```python
from build123d import *

# Parameters (mm, degrees)
F0_W         = 3.3528
F0_H         = 2.5146
F0_R         = 0.80645
F0_W_2       = 6.35
F0_H_2       = 10.7442
F1_DEPTH     = 3.048
F2_W         = 2.54
F2_H         = 10.7442
F2_W_2       = 22.86
F2_H_2       = 7.9502
F3_DEPTH     = 1.27
F4_W         = 6.35
F4_H         = 5.715
F5_DEPTH     = 2.54
F6_R         = 0.79375
F7_DEPTH     = 10.7452
F8_DEPTH     = 0.508
F9_W         = 3.81
F9_H         = 2.5146
F10_DEPTH    = 0.762
F11_T1_DEPTH = 10.445747458
F11_T3_DEPTH = 10.445747458
F11_T5_DEPTH = 12.6746
F11_T7_DEPTH = 12.6746
F12_R        = 0.381
F13_DEPTH    = 1.397


# Not quite as in the source:
# - a fillet or chamfer that OpenCascade refuses, or shapes differently, is made with other operations: its cross-section is extruded or revolved along the edge and cut away or added
# - a feature names something its author has since deleted; it is built from what else it names


with BuildPart() as f1:
    # F0 (on Top) → F1 (new body)
    with BuildSketch(Plane.XY):
        with Locations((-12.8524, 4.1148)):
            Rectangle(F0_W, F0_H)
        with Locations((-12.8524, -4.1148)):
            Rectangle(F0_W, F0_H)
        Polygon((14.478, -5.3721), (14.478, 5.3721), (-11.176, 5.3721), (-11.176, 2.8575), (-11.176, -2.8575), (-11.176, -5.3721), align=None)
        with Locations((-7.366, 0)):
            Circle(F0_R, mode=Mode.SUBTRACT)
        with BuildLine():
            ThreePointArc((-1.7885716042, 1.644670926), (-2.2375844102, 2.728683732), (-1.1535716042, 2.279670926))
            Line((-1.1535716042, 2.279670926), (1.1535716042, 2.279670926))
            ThreePointArc((1.1535716042, 2.279670926), (2.2375844102, 2.728683732), (1.7885716042, 1.644670926))
            Line((1.7885716042, 1.644670926), (1.7885716042, 0.635))
            ThreePointArc((1.7885716042, 0.635), (2.4235716042, 0), (1.7885716042, -0.635))
            Line((1.7885716042, -0.635), (1.7885716042, -1.644670926))
            ThreePointArc((1.7885716042, -1.644670926), (2.2375844102, -2.728683732), (1.1535716042, -2.279670926))
            Line((1.1535716042, -2.279670926), (-1.1535716042, -2.279670926))
            ThreePointArc((-1.1535716042, -2.279670926), (-2.2375844102, -2.728683732), (-1.7885716042, -1.644670926))
            Line((-1.7885716042, -1.644670926), (-1.7885716042, -0.635))
            ThreePointArc((-1.7885716042, -0.635), (-2.4235716042, 0), (-1.7885716042, 0.635))
            Line((-1.7885716042, 0.635), (-1.7885716042, 1.644670926))
        make_face(mode=Mode.SUBTRACT)
        with Locations((10.668, 0)):
            Circle(F0_R, mode=Mode.SUBTRACT)
        with Locations((17.653, 0)):
            Rectangle(F0_W_2, F0_H_2)
    extrude(amount=F1_DEPTH)

    # F2 (on face) → F3 (cut)
    with BuildSketch(Plane.XY.offset(3.048)):
        with Locations((19.558, 0)):
            Rectangle(F2_W, F2_H)
        with Locations((1.651, 0)):
            Rectangle(F2_W_2, F2_H_2)
    extrude(amount=-F3_DEPTH, mode=Mode.SUBTRACT)

    # F4 (on face) → F5 (cut)
    with BuildSketch(Plane.XY.offset(3.048)):
        with Locations((17.653, 0)):
            Rectangle(F4_W, F4_H)
    extrude(amount=-F5_DEPTH, mode=Mode.SUBTRACT)

    # F6 (on face) → F7 (cut, through all)
    with BuildSketch(Plane.XZ.offset(5.3721)):
        with Locations((-12.827, 1.524)):
            Circle(F6_R)
        with Locations((16.2306, 2.159)):
            Circle(F6_R)
    extrude(amount=-F7_DEPTH, mode=Mode.SUBTRACT)

    # F8 (cut): a face of the model
    f8_faces = [f1.faces().sort_by_distance(p)[0] for p in [
        (-9.5369699853, 0, 1.778),
    ]]
    extrude(f8_faces, amount=-F8_DEPTH, mode=Mode.SUBTRACT)

    # F9 (on face) → F10 (join)
    with BuildSketch(Plane.XY.offset(3.048)):
        with Locations((16.383, 4.1148)):
            Rectangle(F9_W, F9_H)
        with Locations((16.383, -4.1148)):
            Rectangle(F9_W, F9_H)
    extrude(amount=F10_DEPTH)

    # F11: fillet of radius 2.032 on 4 edges, made by hand

    # F11_s2 → F11_t1 (cut)
    with BuildSketch(Plane.XZ.offset(-1.108073729)):
        with BuildLine():
            ThreePointArc((16.0642294916, 3.81), (15.1843476813, 3.6096200479), (14.478, 3.048))
            Line((14.478, 3.048), (14.478, 3.81))
            Line((14.478, 3.81), (16.0642294916, 3.81))
        make_face()
    extrude(amount=F11_T1_DEPTH, mode=Mode.SUBTRACT)

    # F11_s4 → F11_t3 (cut)
    with BuildSketch(Plane.XZ.offset(-9.337673729)):
        with BuildLine():
            ThreePointArc((16.0642294916, 3.81), (15.1843476813, 3.6096200479), (14.478, 3.048))
            Line((14.478, 3.048), (14.478, 3.81))
            Line((14.478, 3.81), (16.0642294916, 3.81))
        make_face()
    extrude(amount=F11_T3_DEPTH, mode=Mode.SUBTRACT)

    # F11_s6 → F11_t5 (cut)
    with BuildSketch(Plane.XZ.offset(-10.4521)):
        with BuildLine():
            ThreePointArc((18.288, 1.778), (17.6928409794, 3.2148409794), (16.256, 3.81))
            Line((16.256, 3.81), (18.288, 3.81))
            Line((18.288, 3.81), (18.288, 1.778))
        make_face()
    extrude(amount=F11_T5_DEPTH, mode=Mode.SUBTRACT)

    # F11_s8 → F11_t7 (cut)
    with BuildSketch(Plane.XZ.offset(-2.2225)):
        with BuildLine():
            ThreePointArc((18.288, 1.778), (17.6928409794, 3.2148409794), (16.256, 3.81))
            Line((16.256, 3.81), (18.288, 3.81))
            Line((18.288, 3.81), (18.288, 1.778))
        make_face()
    extrude(amount=F11_T7_DEPTH, mode=Mode.SUBTRACT)

    # F12 (on face) → F13 (cut, through all)
    with BuildSketch(Plane(origin=(-11.176, 0, 0), x_dir=(0, -1, 0), z_dir=(-1, 0, 0))):
        with Locations((-0.9525, 1.9129452994)):
            Circle(F12_R)
    extrude(amount=-F13_DEPTH, mode=Mode.SUBTRACT)


solid = f1.part
```
For this review, take the finished solid that the model builds, in its own axes (mm). A direction names the side the tool comes from. Round coordinates to 2 decimals unless told otherwise and drop trailing zeros. Write each loop counter-clockwise with the first axis right and the second up, starting at its lowest first coordinate (ties: lowest second). Pieces come first, ordered by that corner, then holes. Notation, with made-up numbers: (51, 2) -> (71, 2) arc R21 cw to (71, 12) -> close; hole circle Ø8 at (26, 68). An arc over 180 degrees is marked (long way). One line per question, with ' | ' between items. Start each with the question number.
1) Add section A-A (x = 0.5). Write out the cut boundary in (y, z).
2) Machinability: for faces 4 (the flat face through (13.081, 0, 2)), 5 (the flat face through (-14, 2.858, 2)), 6 (the flat face through (0, 2.28, 1)), 7 (the cylindrical face through (-12.07, -4.13, 1.76)), which of the approach directions +Z, -Z, +X, -X, +Y, -Y give a long, thin tool a straight path to every point of the face, cutting with its end or side? Answer none if there is none.
3) Add section B-B (y = 0). Write out the cut boundary in (x, z).
4) Add section D-D (x = 6). Write out the cut boundary in (y, z), and give its area (3 significant figures).
5) Wall thickness on line 1 along X through (y, z) = (0, 0.35); line 2 along Y through (x, z) = (12, 2.1); line 3 along X through (y, z) = (0.5, 1.1): over which ranges is each line inside the solid? List them lowest first.
6) Mouldability with a two-part tool opening along Y and no side actions: class faces 1 (the flat face through (3, -5.372, 1)), 2 (the cylindrical face through (-2.423, -0.014, 0.626)), 3 (the cylindrical face through (16.988, -4.132, 2.397)) as +Y half, -Y half, draft (parallel to the pull), parting line (faces both ways), or undercut.
7) Add section C-C (z = 3.4). Write out the cut boundary in (x, y), and give its area (3 significant figures).
8) For pin 1 Ø2 at (y, z) = (1, 1.5) entering from -X; pin 2 Ø0.8 at (x, y) = (20, 4) entering from +Z; pin 3 Ø1.3 at (y, z) = (0.5, 2.5) entering from +X, all flat-tipped, find the tip position at first contact; note any pin that passes through.
Reported:
1) outline: (-5.37, 0) -> (-2.28, 0) -> (-2.28, 1.27) -> (-3.98, 1.27) -> (-3.98, 3.05) -> (-5.37, 3.05) -> close; (2.28, 0) -> (5.37, 0) -> (5.37, 3.05) -> (3.98, 3.05) -> (3.98, 1.27) -> (2.28, 1.27) -> close
2) face 4: +Z | face 5: +Z, -Z, -X | face 6: +Z, -Z | face 7: +Y, -Y
3) outline: (-11.18, 0) -> (-8.17, 0) -> (-8.17, 1.27) -> (-9.78, 1.27) -> (-9.78, 3.05) -> (-11.18, 3.05) -> close; (-6.56, 0) -> (-2.42, 0) -> (-2.42, 1.27) -> (-6.56, 1.27) -> close; (2.42, 0) -> (9.86, 0) -> (9.86, 1.27) -> (2.42, 1.27) -> close; (11.47, 0) -> (20.83, 0) -> (20.83, 0.51) -> (14.48, 0.51) -> (14.48, 3.05) -> (13.08, 3.05) -> (13.08, 1.27) -> (11.47, 1.27) -> close
4) outline: (-5.37, 0) -> (5.37, 0) -> (5.37, 3.05) -> (3.98, 3.05) -> (3.98, 1.27) -> (-3.98, 1.27) -> (-3.98, 3.05) -> (-5.37, 3.05) -> close | area: 18.6 mm²
5) line 1: x = -11.18 to -8.17, -6.56 to -2.42, 2.42 to 9.86, 11.47 to 20.83 | line 2: y = -5.37 to -3.98, 3.98 to 5.37 | line 3: x = -11.18 to -8, -6.73 to -2.18, 2.18 to 10.04, 11.3 to 14.48
6) face 1: -Y half | face 2: undercut | face 3: draft
7) outline: (14.84, -5.37) -> (17.48, -5.37) -> (17.48, -2.86) -> (14.84, -2.86) -> close; (14.84, 2.86) -> (17.48, 2.86) -> (17.48, 5.37) -> (14.84, 5.37) -> close | area: 13.3 mm²
8) pin 1: stops at x = -11.18 | pin 2: stops at z = 1.78 | pin 3: stops at x = 14.48
